Part model, mm, in its own coordinate system. A direction names the side the tool comes from. Coordinates: 2 decimals unless noted, no trailing zeros. Write each loop counter-clockwise with the first axis right and the second up, starting at its lowest first coordinate (ties: lowest second). Pieces come first, ordered by that corner, then holes. Notation, with made-up numbers: (-7, -34.75) -> (24, -34.75) arc R26 ccw to (24, -15.75) -> close; hole circle Ø4 at (68.5, 26). An arc over 180 degrees is marked (long way). Write item = value, one per line. Start each with the question number.
Q1. Pin check, flat tips, straight feed: P1, Ø4, axis at y = 12, z = 8, coming from the -X side; P2, Ø6, axis at y = 13.5, z = -77, coming from the +X side. Stop position of each tip, or through.
Q2. Pull direction Y, two halves, no side cores. Call faces 5 (the cylindrical face through (66.377, 2.033, 34.196)), 6 (the flat face through (-47.52, 12.42, 33.21)), 7 (the cylindrical face through (-65.57, 3.06, 38.98)), 8 (the flat face through (0.07, 6.103, -78.589)): released by +Y, released by -Y, zero draft, split by the parting line, or undercut.
Q3. Tool access for faces 1 (the flat face through (-5, 12.4, -57.8)), 2 (the flat face through (47.87, 12.89, 33.41)), 3 (the cylindrical face through (68.807, 4.616, 38.767)), 4 (the flat face through (-68.095, 6.103, 39.234)): list every direction of +Z, -Z, +X, -X, +Y, -Y with a clear straight run to the whole face (end or side of a thin tool).
Q4. Band-saw the part on A-A, the plane z = -64. List the corners of the cut face in (x, y), plus the area to 3 significant figures.
Q5. Band-saw the part on B-B, the plane x = 31. List the corners of the cut face in (y, z), plus the area to 3 significant figures.
Q6. Probe line 1 (Y direction, x = 6, z = -1); line 2 (Z direction, x = -4.5, y = 12.5); line 3 (Z direction, x = -65, y = 3). List the from-to ranges inside material, lowest first.
from build123d import *

# Parameters (mm, degrees)
BOSS_EXTRUDE1_DEPTH      = 15
CUT_EXTRUDE1_REACH       = 103.612
M3_CLEARANCE_HOLE1_D     = 3.6
M3_CLEARANCE_HOLE1_DEPTH = 3
CUT_EXTRUDE2_REACH       = 103.612
CIRPATTERN1_COUNT        = 3
FILLET1_R                = 2
FILLET2_R                = 10
FILLET3_R                = 5


with BuildPart() as part:
    # Sketch2 → Boss-Extrude1 (new body)
    with BuildSketch(Plane(origin=(0, 0, 0), x_dir=(1, 0, 0), z_dir=(0, 1, 0))):
        Polygon((0, 0), (-5, 2.886751346), (-5, 100), (5, 100), (5, 2.886751346), align=None)
    boss_extrude1 = extrude(amount=BOSS_EXTRUDE1_DEPTH)

    # Sketch3 → Cut-Extrude1 (cut, up to next)
    with BuildSketch(Plane(origin=(5, 0, 0), x_dir=(0, 0, -1), z_dir=(1, 0, 0)), mode=Mode.PRIVATE) as cut_extrude1_sk1:
        Polygon((0, 12), (88.803847577, 12), (68.019237886, 0), (0, 0), align=None)
    cut_extrude1_tool1 = extrude(cut_extrude1_sk1.sketch, amount=-CUT_EXTRUDE1_REACH, mode=Mode.PRIVATE) & part.part
    # Sketch3 → Cut-Extrude1 (cut, up to next)
    with BuildSketch(Plane(origin=(5, 0, 0), x_dir=(0, 0, -1), z_dir=(1, 0, 0)), mode=Mode.PRIVATE) as cut_extrude1_sk2:
        Polygon((100, 15), (74.019237886, 0), (100, 0), align=None)
    cut_extrude1_tool2 = extrude(cut_extrude1_sk2.sketch, amount=-CUT_EXTRUDE1_REACH, mode=Mode.PRIVATE) & part.part
    cut_extrude1_1 = cut_extrude1_tool1.solids().sort_by_distance((5, 6.265071, -39.435329))[0]
    add(cut_extrude1_1, mode=Mode.SUBTRACT)
    cut_extrude1_2 = cut_extrude1_tool2.solids().sort_by_distance((5, 5, -91.339746))[0]
    add(cut_extrude1_2, mode=Mode.SUBTRACT)
    cut_extrude1 = cut_extrude1_1 + cut_extrude1_2  # Cut-Extrude1 as one shape, for the pattern or mirror that repeats it

    # M3 Clearance Hole1
    with Locations(Plane(origin=(0, -32.051270189, -18.504809472), x_dir=(1, 0, 0), z_dir=(0, -0.8660254037844417, -0.49999999999999484))):
        with Locations((0, -69.102540378)):
            m3_clearance_hole1 = Hole(M3_CLEARANCE_HOLE1_D / 2, depth=M3_CLEARANCE_HOLE1_DEPTH)

    # Sketch6 → Cut-Extrude2 (cut, up to next)
    with BuildSketch(Plane(origin=(5, 0, 0), x_dir=(0, 0, -1), z_dir=(1, 0, 0)), mode=Mode.PRIVATE) as cut_extrude2_sk1:
        Polygon((74.019237886, 0), (68.019237886, 0), (72.519237886, 2.598076211), align=None)
    cut_extrude2_tool1 = extrude(cut_extrude2_sk1.sketch, amount=-CUT_EXTRUDE2_REACH, mode=Mode.PRIVATE) & part.part
    cut_extrude2 = cut_extrude2_tool1.solids().sort_by_distance((5, 0.866025, -71.519238))[0]
    add(cut_extrude2, mode=Mode.SUBTRACT)

    # CirPattern1: Boss-Extrude1, Cut-Extrude1, M3 Clearance Hole1, Cut-Extrude2 ×3 about axis
    cirpattern1_axis = Axis((0, 0, 0), (0, 1, 0))
    add([boss_extrude1.rotate(cirpattern1_axis, i * 360 / CIRPATTERN1_COUNT) for i in range(1, CIRPATTERN1_COUNT)])
    add([cut_extrude1.rotate(cirpattern1_axis, i * 360 / CIRPATTERN1_COUNT) for i in range(1, CIRPATTERN1_COUNT)], mode=Mode.SUBTRACT)
    add([m3_clearance_hole1.rotate(cirpattern1_axis, i * 360 / CIRPATTERN1_COUNT) for i in range(1, CIRPATTERN1_COUNT)], mode=Mode.SUBTRACT)
    add([cut_extrude2.rotate(cirpattern1_axis, i * 360 / CIRPATTERN1_COUNT) for i in range(1, CIRPATTERN1_COUNT)], mode=Mode.SUBTRACT)

    # Fillet1
    fillet1_edges = [part.edges().sort_by_distance(p)[0] for p in [
        (76.906387956, 12, 44.401923789),
        (-76.906387956, 12, 44.401923789),
        (0, 15, -100),
        (0, 12, -88.803847577),
        (-86.602540378, 15, 50),
        (86.602540378, 15, 50),
    ]]
    fillet(fillet1_edges, radius=FILLET1_R)

    # Fillet2
    fillet2_edges = [part.edges().sort_by_distance(p)[0] for p in [
        (0, 13.5, 5.773502692),
        (-5, 13.5, -2.886751346),
        (5, 13.5, -2.886751346),
    ]]
    fillet(fillet2_edges, radius=FILLET2_R)

    # Fillet3
    fillet3_edges = [part.edges().sort_by_distance(p)[0] for p in [
        (65.953021326, 1.299038106, 32.304491924),
        (60.953021326, 1.299038106, 40.964745962),
        (-60.953021326, 1.299038106, 40.964745962),
        (-65.953021326, 1.299038106, 32.304491924),
        (-5, 1.299038106, -73.269237886),
        (5, 1.299038106, -73.269237886),
    ]]
    fillet(fillet3_edges, radius=FILLET3_R - 0.0001)  # a hair under: the kernel refuses the full size


solid = part.part
Ans:
q1.P1 = -27.32
q1.P2 = 5
q2.face_5 = released by -Y
q2.face_6 = zero draft
q2.face_7 = undercut
q2.face_8 = undercut
q3.face_1 = -Z, -X, +Y, -Y
q3.face_2 = +Z, +Y, -Y
q3.face_3 = none
q3.face_4 = -Z
q4.outline = (-5, 12) -> (5, 12) -> (5, 15) -> (-5, 15) -> close
q4.area = 30.0 mm2
q5.outline = (12, 12.12) -> (15, 12.12) -> (15, 23.67) -> (12, 23.67) -> close
q5.area = 34.6 mm2
q6.line_1 = 12 to 15
q6.line_2 = -94.47 to 8.39
q6.line_3 = 34.16 to 43.3
